```python
from build123d import *

# Parameters (mm, degrees)
BOSS_EXTRUDE1_DEPTH = 1.778
BOSS_EXTRUDE2_DEPTH = 22.86
SKETCH5_R           = 3.556
SKETCH5_W           = 15.748
SKETCH5_H           = 7.112
CUT_EXTRUDE1_DEPTH  = 1.778
FILLET1_R           = 3.556
CUT_EXTRUDE2_DEPTH  = 12.7
CUT_EXTRUDE3_DEPTH  = 12.7
SKETCH9_R           = 3.556
BOSS_EXTRUDE3_DEPTH = 3.81
CUT_EXTRUDE4_DEPTH  = 0.635


with BuildPart() as part:
    # Sketch1 → Boss-Extrude1 (new body)
    with BuildSketch(Plane(origin=(0, 0, 0), x_dir=(1, 0, 0), z_dir=(0, 1, 0))):
        with BuildLine():
            Line((-1.778, 3.3655), (-1.778, 25.8445))
            ThreePointArc((-1.778, 25.8445), (-0.271503729, 29.481503729), (3.3655, 30.988))
            Line((3.3655, 30.988), (27.8765, 30.988))
            ThreePointArc((27.8765, 30.988), (31.513503729, 29.481503729), (33.02, 25.8445))
            Line((33.02, 25.8445), (33.02, 3.3655))
            ThreePointArc((33.02, 3.3655), (31.513503729, -0.271503729), (27.8765, -1.778))
            Line((27.8765, -1.778), (3.3655, -1.778))
            ThreePointArc((3.3655, -1.778), (-0.271503729, -0.271503729), (-1.778, 3.3655))
        make_face()
    extrude(amount=-BOSS_EXTRUDE1_DEPTH)

    # Sketch3 → Boss-Extrude2 (add)
    with BuildSketch(Plane.XZ.offset(1.778)):
        with BuildLine():
            Line((27.8765, 1.778), (3.3655, 1.778))
            ThreePointArc((3.3655, 1.778), (-0.271503729, 0.271503729), (-1.778, -3.3655))
            Line((-1.778, -3.3655), (-1.778, -25.8445))
            ThreePointArc((-1.778, -25.8445), (-0.271503729, -29.481503729), (3.3655, -30.988))
            Line((3.3655, -30.988), (27.8765, -30.988))
            ThreePointArc((27.8765, -30.988), (31.513503729, -29.481503729), (33.02, -25.8445))
            Line((33.02, -25.8445), (33.02, -3.3655))
            ThreePointArc((33.02, -3.3655), (31.513503729, 0.271503729), (27.8765, 1.778))
        make_face()
        with BuildLine():
            Line((0, -3.3655), (0, -25.8445))
            ThreePointArc((0, -25.8445), (0.985732128, -28.224267872), (3.3655, -29.21))
            Line((3.3655, -29.21), (27.8765, -29.21))
            ThreePointArc((27.8765, -29.21), (30.256267872, -28.224267872), (31.242, -25.8445))
            Line((31.242, -25.8445), (31.242, -3.3655))
            ThreePointArc((31.242, -3.3655), (30.256267872, -0.985732128), (27.8765, 0))
            Line((27.8765, 0), (3.3655, 0))
            ThreePointArc((3.3655, 0), (0.985732128, -0.985732128), (0, -3.3655))
        make_face(mode=Mode.SUBTRACT)
    extrude(amount=BOSS_EXTRUDE2_DEPTH)

    # Sketch5 → Cut-Extrude1 (cut)
    with BuildSketch(Plane(origin=(0, 0, 0), x_dir=(1, 0, 0), z_dir=(0, 1, 0))):
        with Locations(Location((24.7269, 5.715, 0), (0, 0, 270))):
            Circle(SKETCH5_R)
        with Locations((11.0109, 5.715)):
            Rectangle(SKETCH5_W, SKETCH5_H)
    extrude(amount=-CUT_EXTRUDE1_DEPTH, mode=Mode.SUBTRACT)

    # Fillet1
    fillet1_edges = [part.edges().sort_by_distance(p)[0] for p in [
        (3.1369, -0.889, -2.159),
        (18.8849, -0.889, -2.159),
        (18.8849, -0.889, -9.271),
        (3.1369, -0.889, -9.271),
    ]]
    fillet(fillet1_edges, radius=FILLET1_R - 0.0001)  # a hair under: the kernel refuses the full size

    # Sketch6 → Cut-Extrude2 (cut)
    with BuildSketch(Plane.ZY.offset(1.778)):
        with BuildLine():
            Line((-11.557, -1.778), (-24.511, -1.778))
            ThreePointArc((-24.511, -1.778), (-25.049815367, -2.001184633), (-25.273, -2.54))
            Line((-25.273, -2.54), (-25.273, -8.128))
            ThreePointArc((-25.273, -8.128), (-25.049815367, -8.666815367), (-24.511, -8.89))
            Line((-24.511, -8.89), (-11.557, -8.89))
            ThreePointArc((-11.557, -8.89), (-11.018184633, -8.666815367), (-10.795, -8.128))
            Line((-10.795, -8.128), (-10.795, -2.54))
            ThreePointArc((-10.795, -2.54), (-11.018184633, -2.001184633), (-11.557, -1.778))
        make_face()
    extrude(amount=-CUT_EXTRUDE2_DEPTH, mode=Mode.SUBTRACT)

    # Sketch7 → Cut-Extrude3 (cut)
    with BuildSketch(Plane(origin=(0, 0, -30.988), x_dir=(-1, 0, 0), z_dir=(0, 0, -1))):
        with BuildLine():
            Line((-23.8125889, -6.35), (-17.4625889, -6.35))
            ThreePointArc((-17.4625889, -6.35), (-16.74416841, -6.64757951), (-16.4465889, -7.366))
            Line((-16.4465889, -7.366), (-16.4465889, -8.128))
            ThreePointArc((-16.4465889, -8.128), (-16.818563288, -9.026025612), (-17.7165889, -9.398))
            Line((-17.7165889, -9.398), (-23.5585889, -9.398))
            ThreePointArc((-23.5585889, -9.398), (-24.456614512, -9.026025612), (-24.8285889, -8.128))
            Line((-24.8285889, -8.128), (-24.8285889, -7.366))
            ThreePointArc((-24.8285889, -7.366), (-24.53100939, -6.64757951), (-23.8125889, -6.35))
        make_face()
    cut_extrude3 = extrude(amount=-CUT_EXTRUDE3_DEPTH, mode=Mode.SUBTRACT)

    # Mirror1: Cut-Extrude3 across plane
    add(cut_extrude3.mirror(Plane(origin=(1.016, 0, 1.016), x_dir=(-0.7071067811865437, 0, 0.7071067811865512), z_dir=(-0.7071067811865512, 0, -0.7071067811865438))), mode=Mode.SUBTRACT)

    # Sketch9 → Boss-Extrude3 (add)
    with BuildSketch(Plane.XZ.offset(1.778)):
        with BuildLine():
            Line((6.6929, -10.541), (15.3289, -10.541))
            ThreePointArc((15.3289, -10.541), (18.327432056, -9.496412634), (20.0279, -6.814852263))
            ThreePointArc((20.0279, -6.814852263), (29.5529, -5.715), (20.0279, -4.615147737))
            ThreePointArc((20.0279, -4.615147737), (18.327432056, -1.933587366), (15.3289, -0.889))
            Line((15.3289, -0.889), (6.6929, -0.889))
            ThreePointArc((6.6929, -0.889), (3.280402674, -2.302502674), (1.8669, -5.715))
            ThreePointArc((1.8669, -5.715), (3.280402674, -9.127497326), (6.6929, -10.541))
        make_face()
        with Locations(Location((24.7269, -5.715, 0), (0, 0, 90))):
            Circle(SKETCH9_R, mode=Mode.SUBTRACT)
        with BuildLine():
            Line((6.6929, -9.271), (15.3289, -9.271))
            ThreePointArc((15.3289, -9.271), (17.843371714, -8.229471714), (18.8849, -5.715))
            ThreePointArc((18.8849, -5.715), (17.843371714, -3.200528286), (15.3289, -2.159))
            Line((15.3289, -2.159), (6.6929, -2.159))
            ThreePointArc((6.6929, -2.159), (4.178428286, -3.200528286), (3.1369, -5.715))
            ThreePointArc((3.1369, -5.715), (4.178428286, -8.229471714), (6.6929, -9.271))
        make_face(mode=Mode.SUBTRACT)
    extrude(amount=BOSS_EXTRUDE3_DEPTH)

    # Sweep1: sweep along a path in Sketch12
    with BuildLine(Plane.XZ.offset(24.638)) as sweep1_path:
        Line((31.242, -25.8445), (31.242, -3.3655))
        ThreePointArc((31.242, -3.3655), (30.256267872, -0.985732128), (27.8765, 0))
        Line((27.8765, 0), (3.3655, 0))
        ThreePointArc((3.3655, 0), (0.985732128, -0.985732128), (0, -3.3655))
        Line((0, -3.3655), (0, -25.8445))
        ThreePointArc((0, -25.8445), (0.985732128, -28.224267872), (3.3655, -29.21))
        Line((3.3655, -29.21), (27.8765, -29.21))
        ThreePointArc((27.8765, -29.21), (30.256267872, -28.224267872), (31.242, -25.8445))
    # Sketch11 → Sweep1 (sweep)
    with BuildSketch(Plane(origin=(0, 0, -9.652), x_dir=(-1, 0, 0), z_dir=(0, 0, -1))):
        Polygon((1.778, -24.638), (0, -24.638), (0.143040428, -26.272959572), align=None)
    sweep(path=sweep1_path.line)

    # Sweep2: sweep along a path in Sketch14
    with BuildLine(Plane(origin=(0, -19.812, 0), x_dir=(-1, 0, 0), z_dir=(0, -1, 0))) as sweep2_path:
        Line((-13.282231977, 29.21), (-3.3655, 29.21))
        ThreePointArc((-3.3655, 29.21), (-0.985732128, 28.224267872), (0, 25.8445))
        Line((0, 25.8445), (0, 3.3655))
        ThreePointArc((0, 3.3655), (-0.985732128, 0.985732128), (-3.3655, 0))
        Line((-3.3655, 0), (-27.8765, 0))
        ThreePointArc((-27.8765, 0), (-30.256267872, 0.985732128), (-31.242, 3.3655))
        Line((-31.242, 3.3655), (-31.242, 11.366960451))
    # Sketch15 → Sweep2 (sweep)
    with BuildSketch(Plane(origin=(13.282231977, 0, 0), x_dir=(0, 0, -1), z_dir=(1, 0, 0))):
        Polygon((29.21, -19.812), (29.21, -18.034), (28.448, -18.796), (28.448, -19.812), align=None)
    sweep(path=sweep2_path.line)

    # Sketch16 → Cut-Extrude4 (cut)
    with BuildSketch(Plane.XY.offset(1.778)):
        Polygon((23.045, -17.599), (23.045, -14.639), (21.925, -14.639), (21.925, -9.999), (23.045, -9.999), (23.045, -7.039), (17.493, -7.039), (17.493, -9.999), (18.613, -9.999), (18.613, -13.007), (15.621, -8.912684211), (12.629, -13.007), (12.629, -9.999), (13.749, -9.999), (13.749, -7.039), (8.197, -7.039), (8.197, -9.999), (9.317, -9.999), (9.317, -14.639), (8.197, -14.639), (8.197, -17.599), (12.581, -17.599), (15.621, -13.439), (18.661, -17.599), align=None)
    extrude(amount=-CUT_EXTRUDE4_DEPTH, mode=Mode.SUBTRACT)


solid = part.part
```
Can you work these out from the model? Positions are in its coordinate system, mm. A direction names the side the tool comes from. Coordinates: 2 decimals unless noted, no trailing zeros. Order: outer loops, then holes, each group sorted by start corner. A loop starts at its lowest first (then second) coordinate and runs counter-clockwise, first axis right, second up. Notation, with made-up numbers: (-7, -35) -> (22, -35) arc R20 cw to (22, -9) -> close; hole circle Ø2 at (-19.5, 10.25). An arc over 180 degrees is marked (long way). Write each question's results on one line, items separated by ' | '.
Item 1: I want a section at B-B, the plane y = -21.5. Write out the boundary of the cut face in (x, z).
Results are:
outline: (-1.78, -25.84) arc R5.14 ccw to (3.37, -30.99) -> (27.88, -30.99) arc R5.14 ccw to (33.02, -25.84) -> (33.02, -3.37) arc R5.14 ccw to (27.88, 1.78) -> (3.37, 1.78) arc R5.14 ccw to (-1.78, -3.37) -> close; hole (0, -25.84) arc R3.37 ccw to (3.37, -29.21) -> (27.88, -29.21) arc R3.37 ccw to (31.24, -25.84) -> (31.24, -3.37) arc R3.37 ccw to (27.88, 0) -> (3.37, 0) arc R3.37 ccw to (0, -3.37) -> close
Item 2: I want a section at C-C, the plane z = -12. Write out the boundary of the cut face in (x, y).
Results are:
outline: (-1.78, -24.64) -> (-0.14, -26.27) -> (0, -24.64) -> (0, -19.81) -> (0.76, -19.81) -> (0.76, -18.8) -> (0, -18.03) -> (0, -8.89) -> (-1.78, -8.89) -> close; (-1.78, -1.78) -> (31.24, -1.78) -> (31.24, -24.64) -> (31.39, -26.27) -> (33.02, -24.64) -> (33.02, 0) -> (-1.78, 0) -> close
Item 3: I'm going to push flat-ended pins straight in: pin 1 Ø0.9 at (x, z) = (22, -30.5) entering from -Y; pin 2 Ø0.7 at (y, z) = (-8.5, 1.5) entering from +X; pin 3 Ø6 at (x, z) = (22, -13) entering from -Y. Where does each tip first touch, or does it pass through?
Results are:
pin 1: y = -25.58 | pin 2: x = 30.34 | pin 3: y = -5.59
Item 4: Which directions (+Z, -Z, +X, -X, +Y, -Y) give clear straight access to the entire face, cutting with the end or side of a thin tool? Please do faces 5 (the face through (30.28, -9.79, -1.01)), 6 (the face through (17.816, -0.901, -8.257)), 7 (the face through (0.96, -22.19, -28.2)).
Results are:
face 5: none | face 6: +Y, -Y | face 7: -Y
Item 5: If I drill on line 1 along X through (y, z) = (-5.75, -8); line 2 along Z through (x, y) = (15.5, -13.5); line 3 along Z through (x, y) = (14, -16.25), over which ranges is the centre line in solid material (lowest first)?
Results are:
line 1: -1.78 to 0, 31.24 to 33.02 | line 2: -30.99 to -29.21, 0 to 1.14 | line 3: -30.99 to -29.21, 0 to 1.78
Item 6: If we mould it in two halves opening along Y, with no side actions, what happens to faces 1 (the face through (17.14, -10.99, 1.46)), 2 (the face through (30.783, -25.626, -28.815)), 3 (the face through (30.48, -19, -7)), 4 (the face through (31.242, -13, -15))? For each: +Y half, -Y half, draft (parallel to the pull), parting line (faces both ways), or undercut.
Results are:
face 1: undercut | face 2: -Y half | face 3: draft | face 4: undercut
Item 7: I want a section at A-A, the plane z = -20.5. Write out the boundary of the cut face in (x, y), then the cut area to 3 significant figures.
Results are:
outline: (-1.78, -24.64) -> (-0.14, -26.27) -> (0, -24.64) -> (0, -19.81) -> (0.76, -19.81) -> (0.76, -18.8) -> (0, -18.03) -> (0, -8.89) -> (-1.78, -8.89) -> close; (-1.78, -1.78) -> (31.24, -1.78) -> (31.24, -6.35) -> (33.02, -6.35) -> (33.02, 0) -> (-1.78, 0) -> close; (31.24, -24.64) -> (31.39, -26.27) -> (33.02, -24.64) -> (33.02, -9.4) -> (31.24, -9.4) -> close | area: 129 mm²
Item 8: I want a section at D-D, the plane x = 27. Write out the boundary of the cut face in (y, z), then the cut area to 3 significant figures.
Results are:
outline: (-26.27, -29.35) -> (-24.64, -30.99) -> (0, -30.99) -> (0, -8.45) -> (-5.59, -8.45) -> (-5.59, -9.97) -> (-1.78, -9.97) -> (-1.78, -29.21) -> (-24.64, -29.21) -> close; (-26.27, 0.14) -> (-24.64, 0) -> (-19.81, 0) -> (-19.81, -0.76) -> (-18.8, -0.76) -> (-18.03, 0) -> (-1.78, 0) -> (-1.78, -1.46) -> (-5.59, -1.46) -> (-5.59, -2.98) -> (0, -2.98) -> (0, 1.78) -> (-24.64, 1.78) -> close | area: 145 mm²
